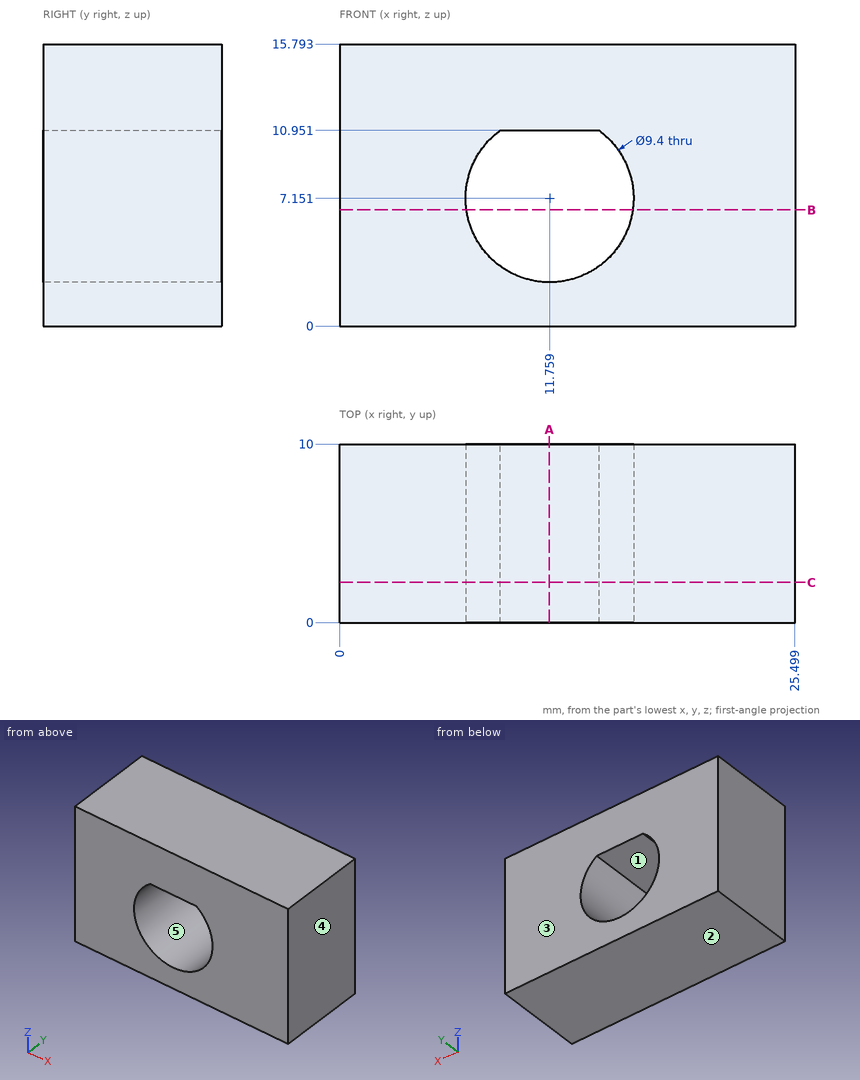
Part print with two shaded views. Sizes in mm from the minimum x, y, z corner. A direction names the side the tool comes from. Round coordinates to 2 decimals unless told otherwise and drop trailing zeros. Order: outer loops, then holes, each group sorted by start corner. A loop starts at its lowest first (then second) coordinate and runs counter-clockwise, first axis right, second up. Notation, with made-up numbers: M 3.5,-31 L 24.5,-31 A15 ccw 24.5,-16 Z; hole C 19.25,-36 d6. An arc over 180 degrees is marked long. Use CSV: the item, a comma, the result in double quotes. Start each with the question number.
(1) Mould opens along X. For the marked faces 3, 4 and 5 say: +X half, -X half, draft (parallel to the pull), parting line (faces both ways), or undercut.
(2) Cut at C-C on y = 2.25. List the corners of the cut face in (x, z) (1 decimal).
(3) Tool access for the marked faces 1 and 2: list every direction of +Z, -Z, +X, -X, +Y, -Y with a clear straight run to the whole face (end or side of a thin tool).
(4) Cut at B-B on z = 6.5. List the corners of the cut face in (x, y) (1 decimal), then the cut area to 3 significant figures.
(5) Drill centre lines: probe 1 along X at (y, z) = (9.25, 3.5); probe 2 along Z at (x, y) = (8, 7.5) (1 decimal); probe 3 along Z at (x, y) = (12.75, 2.25). Where is each one in solid material? Low to high.
(6) Cut at A-A on x = 11.75. List the corners of the cut face in (y, z).
Findings:
1,face 3,"draft"
1,face 4,"+X half"
1,face 5,"undercut"
2,outline,"M 0,0 L 25.5,0 L 25.5,15.8 L 0,15.8 Z; hole M 9,11 A4.7 ccw long 14.5,11 Z"
3,face 1,"+Y, -Y"
3,face 2,"-Z, +X, -X, +Y, -Y"
4,outline,"M 0,0 L 7.1,0 L 7.1,10 L 0,10 Z; M 16.4,0 L 25.5,0 L 25.5,10 L 16.4,10 Z"
4,area,"162 mm^2"
5,probe 1,"x = 0 to 8.8, 14.72 to 25.5"
5,probe 2,"z = 0 to 4.3, 10 to 15.8"
5,probe 3,"z = 0 to 2.56, 10.95 to 15.79"
6,outline,"M 0,0 L 10,0 L 10,2.45 L 0,2.45 Z; M 0,10.95 L 10,10.95 L 10,15.79 L 0,15.79 Z"
